Build history of the part. All positions in model axes, mm. A direction names the side the tool comes from. Round coordinates to 2 decimals unless told otherwise and drop trailing zeros. Write each loop counter-clockwise with the first axis right and the second up, starting at its lowest first coordinate (ties: lowest second). Pieces come first, ordered by that corner, then holes. Notation, with made-up numbers: M -21,-10.5 L -9,-10.5 A24 cw -9,10.5 Z; hole C 14,80 d3. An arc over 180 degrees is marked long. Write item = value, one per line. Start each with the question number.
Q1. Band-saw the part on A-A on y = 0. Write the cut outline in (x, z) (3 decimals).
Q2. Drop flat-ended pins along their axis: P1, Ø10, axis at x = 17.5, z = 20.5, coming from the +Y side; P2, Ø5, axis at x = 7, y = -1.5, coming from the -Z side; P3, Ø8, axis at x = 10, z = 3, coming from the +Y side; P4, Ø2, axis at y = 6.5, z = 16.5, coming from the -X side. Give the stop position or say it passes through.
Q3. Tool access for faces 1 (the flat face through (-8, 2.241, 13)), 2 (the cylindrical face through (11.47, 0.41, 12.52)), 3 (the flat face through (-8, -2.241, 13)): list every direction of +Z, -Z, +X, -X, +Y, -Y with a clear straight run to the whole face (end or side of a thin tool).
Q4. Band-saw the part on D-D on x = -13.5. Write the cut outline in (y, z), plus the area to 3 significant figures.
Q5. Pull direction X, two halves, no side cores. Call faces 4 (the cylindrical face through (-31.164, 0.059, 12.522)), 5 (the cylindrical face through (27.051, 8.886, 12.522)), 6 (the cylindrical face through (21.594, -0.208, 12.522)), 7 (the flat face through (3, 0, 0)): released by +X, released by -X, zero draft, split by the parting line, or undercut.
Q6. Band-saw the part on C-C on y = -4. Write the cut outline in (x, z), plus the area to 3 significant figures.
Q7. Band-saw the part on B-B on z = 3.25. Write the cut outline in (x, y) (3 decimals).
Q8. Probe L1, parallel to X at y = -1, z = 17 (3 decimals); L2, parallel to Y at x = -10.5, z = 12.25; L3, parallel to X at y = -0.25, z = 4.5 (3 decimals). List the from-to ranges inside material, lowest first.
```python
from build123d import *

# Parameters (mm, degrees)
F0_R     = 1.35
F1_DEPTH = 25.4


with BuildPart() as f1:
    # F0 (on Top) → F1 (new body)
    with BuildSketch(Plane.XY):
        with BuildLine():
            Line((-34.925, 2.240668), (-34.925, -2.240668))
            Line((-34.925, -2.240668), (18.702006, -2.240668))
            ThreePointArc((18.702006, -2.240668), (26.892817, -8.880439), (35.663454, -3.027929))
            Line((35.663454, -3.027929), (32.198582, -2.951963))
            ThreePointArc((32.198582, -2.951963), (21.59, 0), (32.198582, 2.951963))
            Line((32.198582, 2.951963), (35.663454, 3.027929))
            ThreePointArc((35.663454, 3.027929), (26.892817, 8.880439), (18.702006, 2.240668))
            Line((18.702006, 2.240668), (-34.925, 2.240668))
        make_face()
        with Locations((-29.815227, 0)):
            Circle(F0_R, mode=Mode.SUBTRACT)
        with Locations((10.184773, 0)):
            Circle(F0_R, mode=Mode.SUBTRACT)
    extrude(amount=F1_DEPTH)


solid = f1.part
```
Conclusion:
q1.outline = M -34.925,0 L -31.165,0 L -31.165,25.4 L -34.925,25.4 Z; M -28.465,0 L 8.835,0 L 8.835,25.4 L -28.465,25.4 Z; M 11.535,0 L 21.59,0 L 21.59,25.4 L 11.535,25.4 Z
q2.P1 = 7.48
q2.P2 = 0
q2.P3 = 2.24
q2.P4 = 20.32
q3.face_1 = +Z, -Z, -X, +Y
q3.face_2 = +Z, -Z
q3.face_3 = +Z, -Z, -X, -Y
q4.outline = M -2.24,0 L 2.24,0 L 2.24,25.4 L -2.24,25.4 Z
q4.area = 114 mm^2
q5.face_4 = undercut
q5.face_5 = split by the parting line
q5.face_6 = undercut
q5.face_7 = zero draft
q6.outline = M 19.37,0 L 23.22,0 L 23.22,25.4 L 19.37,25.4 Z; M 31.39,0 L 35.24,0 L 35.24,25.4 L 31.39,25.4 Z
q6.area = 196 mm^2
q7.outline = M -34.925,-2.241 L 18.702,-2.241 A8.89 ccw 35.663,-3.028 L 32.199,-2.952 A5.715 cw long 32.199,2.952 L 35.663,3.028 A8.89 ccw 18.702,2.241 L -34.925,2.241 Z; hole C -29.815,0 d2.7; hole C 10.185,0 d2.7
q8.L1 = -34.925 to -30.722, -28.908 to 9.278, 11.092 to 21.678
q8.L2 = -2.24 to 2.24
q8.L3 = -34.925 to -31.142, -28.489 to 8.858, 11.511 to 21.595
